Can you work these out from the model? Positions are in its coordinate system, mm. Round coordinates to 2 decimals unless told otherwise and drop trailing zeros. Loops run counter-clockwise (first coordinate to the right, second up) from the corner with the lowest first, then second, coordinate; pieces in that order, holes last. Notation, with made-up numbers: (85, 37) -> (107, 37) arc R29 cw to (107, 74) -> close; hole circle Ø1 at (56.25, 45). An arc over 180 degrees is marked (long way). Answer as a JSON object with one key per item and string values.
```python
from build123d import *

# Parameters (mm, degrees)
SKETCH1_R           = 100
SKETCH1_R_2         = 1.5
BOSS_EXTRUDE1_DEPTH = 4.75


with BuildPart() as part:
    # Sketch1 → Boss-Extrude1 (new body)
    with BuildSketch(Plane.XY):
        with BuildLine():
            Line((-60, -125.000000002), (-60, -131.000000002))
            Line((-60, -131.000000002), (60, -131.000000002))
            Line((60, -131.000000002), (60, -125.000000002))
            Line((60, -125.000000002), (97.529258777, -78.185955788))
            ThreePointArc((97.529258777, -78.185955788), (0, 125), (-97.529258777, -78.185955788))
            Line((-97.529258777, -78.185955788), (-60, -125.000000002))
        make_face()
        Circle(SKETCH1_R, mode=Mode.SUBTRACT)
        with Locations((77.781745931, -77.781745931)):
            Circle(SKETCH1_R_2, mode=Mode.SUBTRACT)
        with Locations((77.781745931, 77.781745931)):
            Circle(SKETCH1_R_2, mode=Mode.SUBTRACT)
        with Locations((0, 110)):
            Circle(SKETCH1_R_2, mode=Mode.SUBTRACT)
        with Locations((-77.781745931, -77.781745931)):
            Circle(SKETCH1_R_2, mode=Mode.SUBTRACT)
        with Locations((-77.781745931, 77.781745931)):
            Circle(SKETCH1_R_2, mode=Mode.SUBTRACT)
        with Locations((110, 0)):
            Circle(SKETCH1_R_2, mode=Mode.SUBTRACT)
        with Locations((-110, 0)):
            Circle(SKETCH1_R_2, mode=Mode.SUBTRACT)
        with Locations((-20, -110)):
            Circle(SKETCH1_R_2, mode=Mode.SUBTRACT)
        with Locations((20, -110)):
            Circle(SKETCH1_R_2, mode=Mode.SUBTRACT)
    extrude(amount=BOSS_EXTRUDE1_DEPTH)


solid = part.part
```
Q1. I want a section at B-B, the plane x = 40.5. Write out the boundary of the cut face in (y, z), then the cut area to 3 significant figures.
Determined:
{"outline": "(-131, 0) -> (-91.43, 0) -> (-91.43, 4.75) -> (-131, 4.75) -> close; (91.43, 0) -> (118.26, 0) -> (118.26, 4.75) -> (91.43, 4.75) -> close", "area": "315 mm²"}
Q2. I want a section at C-C, the plane z = 1.05. Give the number of separate pieces and of enclosed holes in the cut face, then the cut area to 3 significant figures.
Determined:
{"separate pieces": "1", "enclosed holes": "10", "area": "19,300 mm²"}
Q3. We'd pull the mould along X, two halves only. Please class faces 1 (the flat face through (78.5, -101.92, 2.34)), 2 (the cylindrical face through (95.38, 30.04, 2.34)), 3 (the flat face through (27, -97, 0)): pulls with the +X half, pulls with the -X half, needs draft (parallel to the pull), parting line crosses it, or undercut.
Determined:
{"face 1": "pulls with the +X half", "face 2": "undercut", "face 3": "needs draft"}
Q4. If I drill on L1, parallel to X at y = 0.5, z = 1.2; L2, parallel to Y at x = 78, z = 2.65; L3, parallel to X at y = -76.5, z = 3.3, over which ranges is the centre line in solid material (lowest first)? Write a range as [from, to].
Determined:
{"L1": "[-125, -111.41], [-108.59, -100], [100, 108.59], [111.41, 125]", "L2": "[-102.55, -79.27], [-76.3, -62.58], [62.58, 76.3], [79.27, 97.68]", "L3": "[-98.86, -78.56], [-77, -64.4], [64.4, 77], [78.56, 98.86]"}
Q5. I want a section at A-A, the plane y = -25.5. Write out the boundary of the cut face in (x, z).
Determined:
{"outline": "(-122.37, 0) -> (-96.69, 0) -> (-96.69, 4.75) -> (-122.37, 4.75) -> close; (96.69, 0) -> (122.37, 0) -> (122.37, 4.75) -> (96.69, 4.75) -> close"}
Q6. I'm going to push flat-ended pins straight in: pin 1 (1.5 mm diameter, centred on y = 65.5, z = 1, fed in from +X); pin 2 (1.4 mm diameter, centred on y = -127, z = 2.5, fed in from +X). Where does each tip first touch, or does it pass through?
Determined:
{"pin 1": "x = 106.92", "pin 2": "x = 60"}
